```python
from build123d import *

# Parameters (mm, degrees)
F2_W     = 76.2
F2_H     = 50.8
F3_DEPTH = 76.2
F1_W     = 127
F1_H     = 76.2
F4_DEPTH = 25.4
F5_R     = 9.525
F7_DEPTH = 25.4
F6_R     = 9.525
F9_DEPTH = 25.4


with BuildPart() as f3:
    # F2 (on Right) → F3 (new body)
    with BuildSketch(Plane.YZ):
        with Locations((38.1, 25.4)):
            Rectangle(F2_W, F2_H)
    extrude(amount=F3_DEPTH)

    # F1 (on Top) → F4 (join)
    with BuildSketch(Plane.XY):
        with Locations((63.5, 38.1)):
            Rectangle(F1_W, F1_H)
    extrude(amount=F4_DEPTH)

    # F5 (on face) → F7 (cut)
    with BuildSketch(Plane.XY.offset(50.8)):
        with Locations((38.089141, 38.1)):
            Circle(F5_R)
    extrude(amount=-F7_DEPTH, mode=Mode.SUBTRACT)

    # F6 (on face) → F9 (cut)
    with BuildSketch(Plane.YZ.offset(76.2)):
        with Locations((38.1, 37.928037)):
            Circle(F6_R)
    extrude(amount=-F9_DEPTH, mode=Mode.SUBTRACT)


solid = f3.part
```
Model file for the job. Use its own axes, mm. A direction names the side the tool comes from. Coordinates: 2 decimals unless noted, no trailing zeros. Write each loop counter-clockwise with the first axis right and the second up, starting at its lowest first coordinate (ties: lowest second). Pieces come first, ordered by that corner, then holes. Notation, with made-up numbers: (55.5, -21.75) - (110.5, -21.75) arc R25 ccw to (110.5, -8.75) - close; hole circle Ø11 at (78.5, -30). An arc over 180 degrees is marked (long way). One line per question, with ' | ' between items. Start each with the question number.
Q1. Cut at B-B, the plane x = 56. List the corners of the cut face in (y, z) (3 decimals), then the cut area to 3 significant figures.
Q2. 3-axis set-ups, long thin cutter, end or side, ignore diameter. For faces 1 (the face through (38, 38, 25.4)), 2 (the face through (76.2, 29, 44)), 3 (the face through (48, 0, 19)): which of +Z, -Z, +X, -X, +Y, -Y reach the whole face in a straight line?
Q3. Pull direction Z, two halves, no side cores. Call faces 4 (the face through (31.07, 44.54, 38.28)), 5 (the face through (63.678, 31.08, 44.365)), 6 (the face through (46, 46, 50.8)), 7 (the face through (50.8, 38, 38)): pulls with the +Z half, pulls with the -Z half, needs draft (parallel to the pull), parting line crosses it, or undercut.
Q4. Drill centre lines: line 1 (Z direction, x = 62.5, y = 38.1); line 2 (Z direction, x = 103.5, y = 52); line 3 (X direction, y = 69, z = 45.5). Where is each one in solid material? Low to high. Write a range as [from, to].
Q5. Pin check, flat tips, straight feed: pin 1 (25 mm diameter, centred on y = 38.1, z = 37.93, fed in from +X); pin 2 (11.5 mm diameter, centred on x = 38.09, y = 38.1, fed in from +Z); pin 3 (5.5 mm diameter, centred on y = 36.5, z = 36.5, fed in from +X). Stop position of each tip, or through.
Q6. Cut at A-A, the plane y = 38.1. List the corners of the cut face in (x, z).
Q7. Cut at C-C, the plane z = 31.5. List the corners of the cut face in (x, y) (3 decimals).
Q8. Cut at D-D, the plane x = 112. List the corners of the cut face in (y, z).
Answer below:
1) outline: (0, 0) - (76.2, 0) - (76.2, 50.8) - (0, 50.8) - close; hole circle Ø19.05 at (38.1, 37.928) | area: 3,590 mm^2
2) face 1: +Z | face 2: +Z, +X, +Y, -Y | face 3: +Z, -Z, +X, -X, -Y
3) face 4: needs draft | face 5: undercut | face 6: pulls with the +Z half | face 7: undercut
4) line 1: [0, 28.4], [47.45, 50.8] | line 2: [0, 25.4] | line 3: [0, 76.2]
5) pin 1: x = 76.2 | pin 2: z = 25.4 | pin 3: x = 50.8
6) outline: (0, 0) - (127, 0) - (127, 25.4) - (76.2, 25.4) - (76.2, 28.4) - (50.8, 28.4) - (50.8, 47.45) - (76.2, 47.45) - (76.2, 50.8) - (47.61, 50.8) - (47.61, 25.4) - (28.56, 25.4) - (28.56, 50.8) - (0, 50.8) - close
7) outline: (0, 0) - (76.2, 0) - (76.2, 31.071) - (50.8, 31.071) - (50.8, 45.129) - (76.2, 45.129) - (76.2, 76.2) - (0, 76.2) - close; hole circle Ø19.05 at (38.089, 38.1)
8) outline: (0, 0) - (76.2, 0) - (76.2, 25.4) - (0, 25.4) - close
